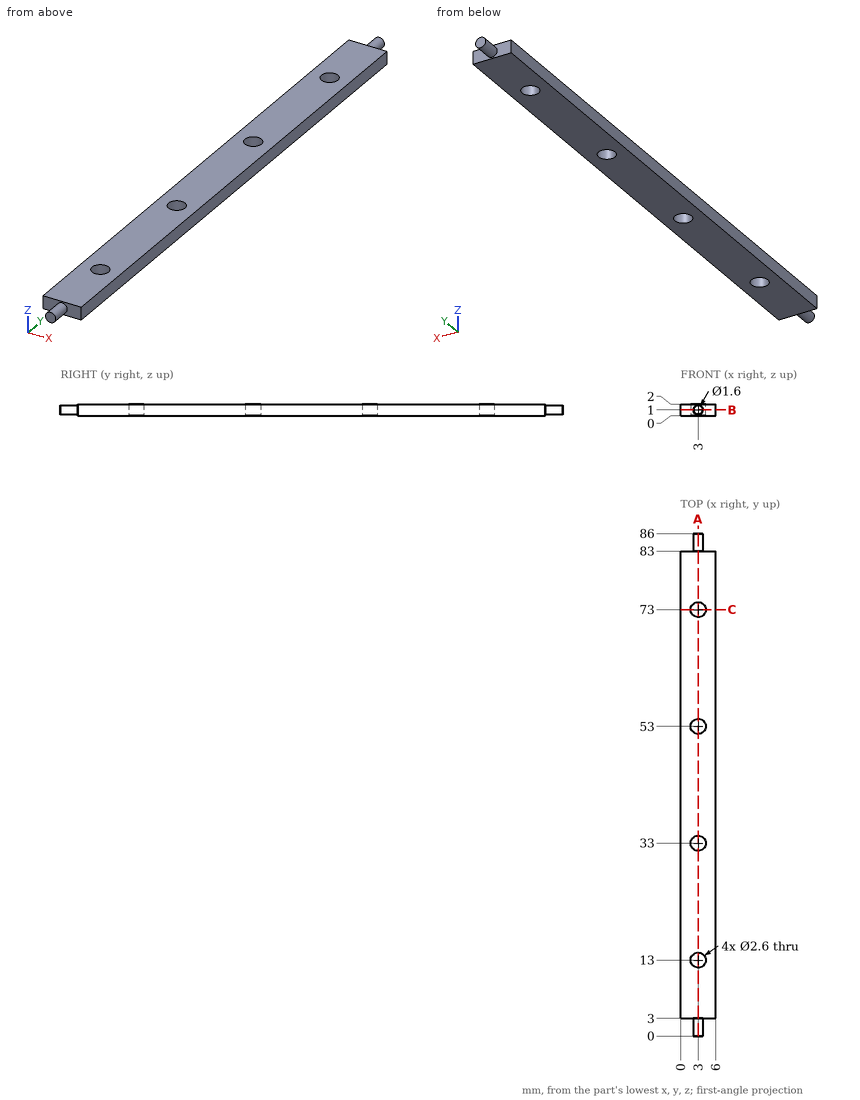
Geometry check sheet. Reference: drawing and pictorial views, mm from the part's lowest x, y, z. Coordinates: 2 decimals unless noted, no trailing zeros. Order: outer loops, then holes, each group sorted by start corner. A loop starts at its lowest first (then second) coordinate and runs counter-clockwise, first axis right, second up. Notation, with made-up numbers: (89, -11) -> (128, -11) arc R25 cw to (128, 20) -> close; hole circle Ø2 at (50, 49.25). An arc over 180 degrees is marked (long way). Use CSV: the item, a comma, the result in double quotes. Start each with the question number.
Q1. Section check B-B, the plane z = 1. Record the cut outline in (x, y), and give its area (3 significant figures).
Q2. Thickness scan on line 1 along Y through (x, z) = (3, 1.65); line 2 along X through (y, z) = (13, 1.1); line 3 along Y through (x, z) = (2.1, 1.6). Record the ranges inside material, lowest first.
Q3. Section check A-A, the plane x = 3. Record the cut outline in (y, z), and give its area (3 significant figures).
Q4. Depth check by flat-ended pin: P1, Ø3, axis at x = 4.5, y = 9, coming from the -Z side; P2, Ø1, axis at x = 4.5, z = 1, coming from the +Y side. Enter the tip coordinate at first touch or a pass-through.
Q5. Section check C-C, the plane y = 73. Record the cut outline in (x, z).
Returned:
1,outline,"(0, 3) -> (2.2, 3) -> (2.2, 0) -> (3.8, 0) -> (3.8, 3) -> (6, 3) -> (6, 83) -> (3.8, 83) -> (3.8, 86) -> (2.2, 86) -> (2.2, 83) -> (0, 83) -> close; hole circle Ø2.6 at (3, 13); hole circle Ø2.6 at (3, 33); hole circle Ø2.6 at (3, 53); hole circle Ø2.6 at (3, 73)"
1,area,"468 mm^2"
2,line 1,"y = 0 to 11.7, 14.3 to 31.7, 34.3 to 51.7, 54.3 to 71.7, 74.3 to 86"
2,line 2,"x = 0 to 1.7, 4.3 to 6"
2,line 3,"y = 3 to 12.06, 13.94 to 32.06, 33.94 to 52.06, 53.94 to 72.06, 73.94 to 83"
3,outline,"(0, 0.2) -> (3, 0.2) -> (3, 0) -> (11.7, 0) -> (11.7, 2) -> (3, 2) -> (3, 1.8) -> (0, 1.8) -> close; (14.3, 0) -> (31.7, 0) -> (31.7, 2) -> (14.3, 2) -> close; (34.3, 0) -> (51.7, 0) -> (51.7, 2) -> (34.3, 2) -> close; (54.3, 0) -> (71.7, 0) -> (71.7, 2) -> (54.3, 2) -> close; (74.3, 0) -> (83, 0) -> (83, 0.2) -> (86, 0.2) -> (86, 1.8) -> (83, 1.8) -> (83, 2) -> (74.3, 2) -> close"
3,area,"149 mm^2"
4,P1,"stops at z = 0"
4,P2,"stops at y = 83"
5,outline,"(0, 0) -> (1.7, 0) -> (1.7, 2) -> (0, 2) -> close; (4.3, 0) -> (6, 0) -> (6, 2) -> (4.3, 2) -> close"
